Design review of the part built by this model. Coordinates are the model's own, in mm. Face numbers are marked on the shaded views. Coordinates: 2 decimals unless noted, no trailing zeros. Loops run counter-clockwise (first coordinate to the right, second up) from the corner with the lowest first, then second, coordinate; pieces in that order, holes last. Notation, with made-up numbers: (33, 31.25) - (42, 31.25) arc R30 ccw to (42, 62.25) - close; hole circle Ø3 at (-30, -18.75). An arc over 180 degrees is marked (long way). Use one line per item in the form item = value. Start each with the question number.
(1) Clearance check with flat-ended pins moving along their axes: pin 1 Ø5 at (x, y) = (18, -9.5) entering from +Z; pin 2 Ø1 at (y, z) = (-17.5, 0.5) entering from +X; pin 3 Ø3 at (y, z) = (21, 3.5) entering from -X. State where each tip first meets the part, or that it passes through.
(2) The part is to be moulded in two halves that separate along X. For the marked faces 1, 2 and 3, say which applies: pulls with the +X half, pulls with the -X half, needs draft (parallel to the pull), parting line crosses it, or undercut.
(3) Add section C-C (z = 3.95). State the section outline as (x, y) points (3 decimals), plus the area to 3 significant figures.
(4) Add section A-A (x = 0). State the section outline as (y, z) points.
(5) For L1, parallel to Y at x = 0, z = 3.65; L2, parallel to Y at x = 0, z = 1.95; L3, parallel to Z at x = -20, y = -9, list the stretches that pass through material, from the lowest coordinate up.
(6) Add section B-B (y = 0). State the section outline as (x, z) points.
(7) Add section D-D (y = -10). Count the separate pieces of the cut face and the enclosed holes in it, plus the area to 3 significant figures.
```python
from build123d import *

# Parameters (mm, degrees)
SKETCH1_R            = 26
BOSS_EXTRUDE1_DEPTH  = 5
M5_CLEARANCE_HOLE1_D = 5
CIRPATTERN1_COUNT    = 3
SKETCH4_R            = 11
CUT_EXTRUDE1_DEPTH   = 5
FILLET1_R            = 0.2
SKETCH5_R            = 5
CUT_EXTRUDE2_DEPTH   = 3


with BuildPart() as part:
    # Sketch1 → Boss-Extrude1 (new body)
    with BuildSketch(Plane.XY):
        Circle(SKETCH1_R)
    extrude(amount=BOSS_EXTRUDE1_DEPTH)

    # M5 Clearance Hole1 (through all)
    with Locations(Plane.XY.offset(5)):
        with Locations((0, 18.75)):
            m5_clearance_hole1 = Hole(M5_CLEARANCE_HOLE1_D / 2)

    # CirPattern1: M5 Clearance Hole1 ×3 about axis
    cirpattern1_axis = Axis((0, 0, 0), (0, 0, 1))
    for i in range(1, CIRPATTERN1_COUNT):
        add(m5_clearance_hole1.rotate(cirpattern1_axis, i * 360 / CIRPATTERN1_COUNT), mode=Mode.SUBTRACT)

    # Sketch4 → Cut-Extrude1 (cut)
    with BuildSketch(Plane.XY.offset(5)):
        Circle(SKETCH4_R)
    extrude(amount=-CUT_EXTRUDE1_DEPTH, mode=Mode.SUBTRACT)

    # Fillet1
    fillet1_edges = [part.edges().sort_by_distance(p)[0] for p in [
        (-26, 0, 0),
        (-26, 0, 5),
    ]]
    fillet(fillet1_edges, radius=FILLET1_R)

    # Sketch5 → Cut-Extrude2 (cut)
    with BuildSketch(Plane.XY.offset(5)):
        with Locations((0, 18.75)):
            Circle(SKETCH5_R)
        with Locations((-16.237976321, -9.375)):
            Circle(SKETCH5_R)
        with Locations((16.237976321, -9.375)):
            Circle(SKETCH5_R)
    extrude(amount=-CUT_EXTRUDE2_DEPTH, mode=Mode.SUBTRACT)


solid = part.part
```
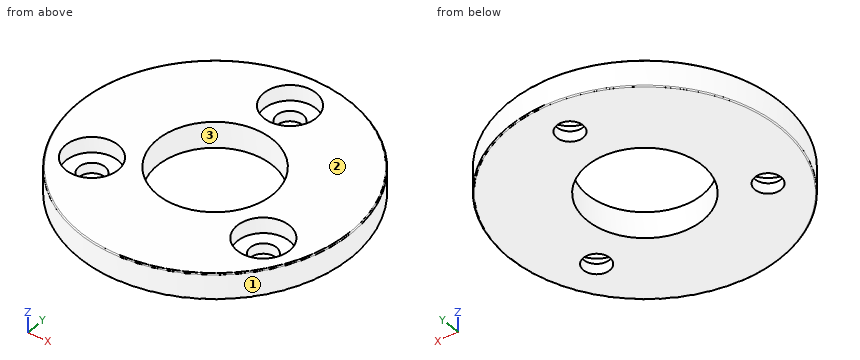
Computed values:
q1.pin_1 = 2
q1.pin_2 = 19.67
q1.pin_3 = -17.2
q2.face_1 = parting line crosses it
q2.face_2 = needs draft
q2.face_3 = undercut
q3.outline = circle Ø52 at (0, 0); hole circle Ø10 at (-16.238, -9.375); hole circle Ø22 at (0, 0); hole circle Ø10 at (0, 18.75); hole circle Ø10 at (16.238, -9.375)
q3.area = 1,510 mm^2
q4.outline = (-26, 0.2) arc R0.2 ccw to (-25.8, 0) - (-11, 0) - (-11, 5) - (-25.8, 5) arc R0.2 ccw to (-26, 4.8) - close; (11, 0) - (16.25, 0) - (16.25, 2) - (13.75, 2) - (13.75, 5) - (11, 5) - close; (21.25, 0) - (25.8, 0) arc R0.2 ccw to (26, 0.2) - (26, 4.8) arc R0.2 ccw to (25.8, 5) - (23.75, 5) - (23.75, 2) - (21.25, 2) - close
q5.L1 = -26 to -11, 11 to 13.75, 23.75 to 26
q5.L2 = -26 to -11, 11 to 16.25, 21.25 to 26
q5.L3 = 0 to 2
q6.outline = (-26, 0.2) arc R0.2 ccw to (-25.8, 0) - (-11, 0) - (-11, 5) - (-25.8, 5) arc R0.2 ccw to (-26, 4.8) - close; (11, 0) - (25.8, 0) arc R0.2 ccw to (26, 0.2) - (26, 4.8) arc R0.2 ccw to (25.8, 5) - (11, 5) - close
q7.separate_pieces = 4
q7.enclosed_holes = 0
q7.area = 115 mm^2
